Here's how the part is built. I have some questions about the finished solid (model axes, mm). A direction names the side the tool comes from. Coordinates: 2 decimals unless noted, no trailing zeros. Loops run counter-clockwise (first coordinate to the right, second up) from the corner with the lowest first, then second, coordinate; pieces in that order, holes last. Notation, with made-up numbers: (80.5, 23) - (133.5, 23) arc R30 cw to (133.5, 57) - close; hole circle Ø8 at (26, 52). An arc over 180 degrees is marked (long way). Use a Markdown table: item, result.
```python
from build123d import *

# Parameters (mm, degrees)
F1_DEPTH = 63.5
F0_W     = 25.4
F0_H     = 12.7
F2_DEPTH = 25.4
F3_DEPTH = 15.875
F5_R     = 5.08


with BuildPart() as f1:
    # F0 (on Front) → F1 (new body, symmetric)
    with BuildSketch(Plane.XZ):
        Polygon((-41.275, -9.525), (41.275, -9.525), (41.275, 9.525), (22.225, 9.525), (-41.275, 9.525), align=None)
    extrude(amount=F1_DEPTH, both=True)

    # F0 (on Front) → F2 (join, symmetric)
    with BuildSketch(Plane.XZ):
        with BuildLine():
            Line((22.225, 9.525), (41.275, 9.525))
            Line((41.275, 9.525), (41.275, 38.1))
            ThreePointArc((41.275, 38.1), (45.92468, 49.32532), (57.15, 53.975))
            Line((57.15, 53.975), (60.325, 53.975))
            Line((60.325, 53.975), (60.325, 66.675))
            Line((60.325, 66.675), (85.725, 66.675))
            Line((85.725, 66.675), (85.725, 73.025))
            Line((85.725, 73.025), (57.15, 73.025))
            ThreePointArc((57.15, 73.025), (32.454296, 62.795704), (22.225, 38.1))
            Line((22.225, 38.1), (22.225, 9.525))
        make_face()
        with Locations((73.025, 60.325)):
            Rectangle(F0_W, F0_H)
    extrude(amount=F2_DEPTH, both=True)

    # F0 (on Front) → F3 (join)
    with BuildSketch(Plane.XZ):
        with BuildLine():
            add(Edge.make_bspline(
                [(-41.275, 9.525), (-8.466667, 30.691667), (25.044836, 75.964727), (57.15, 73.025)],
                knots=[0, 0, 0, 0, 117.131254, 117.131254, 117.131254, 117.131254], degree=3))
            Line((-41.275, 9.525), (22.225, 9.525))
            Line((22.225, 9.525), (22.225, 38.1))
            ThreePointArc((22.225, 38.1), (32.454296, 62.795704), (57.15, 73.025))
        make_face()
    extrude(amount=F3_DEPTH)

    # F0 (on Front) → F4 (revolve)
    with BuildSketch(Plane.XZ):
        Polygon((85.725, 53.975), (60.325, 53.975), (60.325, 38.1), (111.125, 38.1), (111.125, 66.675), (85.725, 66.675), align=None)
    revolve(axis=Axis((60.325, 0, 52.3875), (0, 0, 1)))

    # F5
    f5_edges = [f1.edges().sort_by_distance(p)[0] for p in [
        (41.275, -63.5, 0),
        (-41.275, -63.5, 0),
        (41.275, 63.5, 0),
        (-41.275, 63.5, 0),
    ]]
    fillet(f5_edges, radius=F5_R)


solid = f1.part
```
Q1. If we mould it in two halves opening along Z, with no side actions, what happens to faces 6 (the face through (32, -25.4, 24)), 7 (the face through (-39.8, -62, -0.1)), 8 (the face through (72, 0, 73.025)), 9 (the face through (22.225, -21, 24))? For each: pulls with the +Z half, pulls with the -Z half, needs draft (parallel to the pull), parting line crosses it, or undercut.
Check values:
| item | result |
|---|---|
| face 6 | undercut |
| face 7 | needs draft |
| face 8 | pulls with the +Z half |
| face 9 | undercut |
Q2. I want a section at D-D, the plane y = -42. Write out the boundary of the cut face in (x, z) (3 decimals), then the cut area to 3 significant figures.
Check values:
| item | result |
|---|---|
| outline | (-41.275, -9.525) - (41.275, -9.525) - (41.275, 9.525) - (-41.275, 9.525) - close; (31.748, 38.1) - (88.902, 38.1) - (88.902, 66.675) - (31.748, 66.675) - close |
| area | 3,210 mm^2 |
Q3. I want a section at B-B, the plane z = -2.5. Write out the boundary of the cut face in (x, y) (3 decimals), then the cut area to 3 significant figures.
Check values:
| item | result |
|---|---|
| outline | (-41.275, -58.42) arc R5.08 ccw to (-36.195, -63.5) - (36.195, -63.5) arc R5.08 ccw to (41.275, -58.42) - (41.275, 58.42) arc R5.08 ccw to (36.195, 63.5) - (-36.195, 63.5) arc R5.08 ccw to (-41.275, 58.42) - close |
| area | 10,500 mm^2 |
Q4. Will these pins go through, and if not, where does the flat tip stop? P1, Ø5, axis at x = 39, z = 33.5, coming from the +Y side; P2, Ø3, axis at y = 2, z = 71, coming from the +X side (3 decimals); P3, Ø3, axis at y = 42, z = 39, coming from the +X side.
Check values:
| item | result |
|---|---|
| P1 | y = 25.4 |
| P2 | x = 85.725 |
| P3 | x = 90.99 |
Q5. Which directions (+Z, -Z, +X, -X, +Y, -Y) give clear straight access to the entire face, cutting with the end or side of a thin tool? Please do faces 1 (the face through (-2, 0, 21)), 2 (the face through (108.78, 15.26, 52.59)), 3 (the face through (46.763, -20.704, 71.445)), 4 (the face through (66, -25.4, 70)), 5 (the face through (41.275, -1, 9)).
Check values:
| item | result |
|---|---|
| face 1 | -X, +Y |
| face 2 | +Z |
| face 3 | +Z, -X, -Y |
| face 4 | +Z, +X, -X, -Y |
| face 5 | -Z, +X, +Y, -Y |
Q6. Please list where these lines run through material, in increasing order: L1, parallel to Z at x = 30, y = -31 (3 decimals); L2, parallel to X at y = -16, z = 18.5 (3 decimals); L3, parallel to X at y = -20, z = 8.5 (3 decimals). Write a range as from..to.
Check values:
| item | result |
|---|---|
| L1 | -9.525..9.525, 38.1..66.675 |
| L2 | 22.225..41.275 |
| L3 | -41.275..41.275 |
Q7. I want a section at C-C, the plane y = 14.5. Write out the boundary of the cut face in (x, z) (3 decimals), then the cut area to 3 significant figures.
Check values:
| item | result |
|---|---|
| outline | (-41.275, -9.525) - (41.275, -9.525) - (41.275, 38.1) - (109.012, 38.1) - (109.012, 66.675) - (85.725, 66.675) - (85.725, 73.025) - (57.15, 73.025) arc R34.925 ccw to (37.07, 66.675) - (11.638, 66.675) - (11.638, 38.1) - (22.225, 38.1) - (22.225, 9.525) - (-41.275, 9.525) - close |
| area | 5,170 mm^2 |
Q8. I want a section at A-A, the plane y = -28.5. Write out the boundary of the cut face in (x, z) (3 decimals).
Check values:
| item | result |
|---|---|
| outline | (-41.275, -9.525) - (41.275, -9.525) - (41.275, 9.525) - (-41.275, 9.525) - close; (18.273, 38.1) - (102.377, 38.1) - (102.377, 66.675) - (18.273, 66.675) - close |
